from build123d import *

# Parameters (mm, degrees)
SKETCH1_R           = 1.5
SKETCH1_R_2         = 1
BOSS_EXTRUDE1_DEPTH = 3
FILLET1_R           = 5
FILLET2_R           = 3.5
FILLET3_R           = 1.5


with BuildPart() as part:
    # Sketch1 → Boss-Extrude1 (new body)
    with BuildSketch(Plane.XY):
        Polygon((0, 0), (39, 0), (39, 8.610580904), (15.926488874, 8.610580904), (15.926488874, 14.070663707), (7.926488874, 14.070663707), (7.926488874, 8), (0, 8), align=None)
        with Locations((4.5, 4)):
            Circle(SKETCH1_R, mode=Mode.SUBTRACT)
        with Locations((34.5, 4)):
            Circle(SKETCH1_R, mode=Mode.SUBTRACT)
        with Locations((12.926488874, 11.070663707)):
            Circle(SKETCH1_R_2, mode=Mode.SUBTRACT)
    extrude(amount=BOSS_EXTRUDE1_DEPTH)

    # Fillet1
    # the kernel refuses this fillet: 5 mm, written as the material it takes off along each edge
    with BuildSketch(Plane(origin=(39, 8.610580904, -12.5), x_dir=(0, -1, 0), z_dir=(0, 0, 1)), Plane(origin=(39, 0, -12.5), x_dir=(-1, 0, 0), z_dir=(0, 0, 1)), Plane(origin=(0, 8, -12.5), x_dir=(1, 0, 0), z_dir=(0, 0, 1))) as fillet1_piece_1:
        with BuildLine():
            CenterArc((FILLET1_R, -FILLET1_R), FILLET1_R, 90, 90)
            Line((0, -FILLET1_R), (0, 0))
            Line((0, 0), (FILLET1_R, 0))
        make_face()
    extrude(amount=28, mode=Mode.SUBTRACT)
    with BuildSketch(Plane(origin=(0, 0, -12.5), x_dir=(1, 0, 0), z_dir=(0, 0, 1))) as fillet1_piece_2:
        with BuildLine():
            CenterArc((FILLET1_R, FILLET1_R), FILLET1_R, 180, 90)
            Line((0, FILLET1_R), (0, 0))
            Line((0, 0), (FILLET1_R, 0))
        make_face()
    extrude(amount=28, mode=Mode.SUBTRACT)

    # Fillet2
    fillet2_edges = [part.edges().sort_by_distance(p)[0] for p in [
        (7.926488874, 14.070663707, 1.5),
        (15.926488874, 14.070663707, 1.5),
    ]]
    fillet(fillet2_edges, radius=FILLET2_R)

    # Fillet3
    fillet3_edges = [part.edges().sort_by_distance(p)[0] for p in [
        (7.926488874, 8, 1.5),
        (15.926488874, 8.610580904, 1.5),
    ]]
    fillet(fillet3_edges, radius=FILLET3_R)


solid = part.part
The model under review builds one solid part; all positions refer to its coordinate system, in mm. A direction names the side the tool comes from. Round coordinates to 2 decimals unless told otherwise and drop trailing zeros. Write each loop counter-clockwise with the first axis right and the second up, starting at its lowest first coordinate (ties: lowest second). Pieces come first, ordered by that corner, then holes. Notation, with made-up numbers: (24, 52) -> (55, 52) arc R17 ccw to (55, 79) -> close; hole circle Ø5 at (-36.5, -5). An arc over 180 degrees is marked (long way). Answer as a JSON object with one key per item and string values.
1. We need section C-C on x = 19. State the section outline as (y, z) points.
Results found:
{"outline": "(0, 0) -> (8.61, 0) -> (8.61, 3) -> (0, 3) -> close"}
2. Clearance check with flat-ended pins moving along their axes: pin 1 (2.5 mm diameter, centred on x = 12.93, y = 11.07, fed in from -Z); pin 2 (0.5 mm diameter, centred on y = 10, z = 2, fed in from -X); pin 3 (1.5 mm diameter, centred on y = 2.5, z = 2, fed in from -X); pin 4 (1.1 mm diameter, centred on x = 5.5, z = 1.5, fed in from +Y). State where each tip first meets the part, or that it passes through.
Results found:
{"pin 1": "stops at z = 0", "pin 2": "stops at x = 7.93", "pin 3": "stops at x = 0.32", "pin 4": "stops at y = 8"}
3. The part is to be moulded in two halves that separate along Y. For faces 1 (the face through (13.85, 10.69, 1.48)), 2 (the face through (7.5, 8.45, 1.52)), 3 (the face through (7.926, 10, 1)), say which applies: pulls with the +Y half, pulls with the -Y half, needs draft (parallel to the pull), parting line crosses it, or undercut.
Results found:
{"face 1": "undercut", "face 2": "pulls with the +Y half", "face 3": "needs draft"}
4. Machinability: for faces 4 (the face through (19, 6, 3)), 5 (the face through (6, 8, 1)), 6 (the face through (26, 8.611, 1)), which of the approach directions +Z, -Z, +X, -X, +Y, -Y give a long, thin tool a straight path to every point of the face, cutting with its end or side? Answer none if there is none.
Results found:
{"face 4": "+Z, +X, -X, +Y, -Y", "face 5": "+Z, -Z, -X, +Y", "face 6": "+Z, -Z, +X, +Y"}
5. We need section A-A on x = 4.5. State the section outline as (y, z) points, and give its area (3 significant figures).
Results found:
{"outline": "(0.03, 0) -> (2.5, 0) -> (2.5, 3) -> (0.03, 3) -> close; (5.5, 0) -> (7.97, 0) -> (7.97, 3) -> (5.5, 3) -> close", "area": "14.8 mm^2"}
6. We need section B-B on z = 0.6. State the section outline as (x, y) points, and give its area (3 significant figures).
Results found:
{"outline": "(0.1, 4) arc R5 ccw to (5, 0) -> (34, 0) arc R5 ccw to (38.95, 4.31) arc R5 ccw to (34, 8.61) -> (17.43, 8.61) arc R1.5 cw to (15.93, 10.11) -> (15.93, 10.57) arc R3.5 ccw to (12.43, 14.07) -> (11.43, 14.07) arc R3.5 ccw to (7.93, 10.57) -> (7.93, 9.5) arc R1.5 cw to (6.43, 8) -> (5, 8) arc R5 ccw to start; hole circle Ø3 at (4.5, 4); hole circle Ø2 at (12.93, 11.07); hole circle Ø3 at (34.5, 4)", "area": "332 mm^2"}
7. We need section D-D on x = 34.5. State the section outline as (y, z) points, and give its area (3 significant figures).
Results found:
{"outline": "(0.03, 0) -> (2.5, 0) -> (2.5, 3) -> (0.03, 3) -> close; (5.5, 0) -> (8.59, 0) -> (8.59, 3) -> (5.5, 3) -> close", "area": "16.7 mm^2"}
8. To check wall thickness, follow line 1 along X through (y, z) = (3, 2.1); line 2 along Y through (x, z) = (32, 1.9); line 3 along Y through (x, z) = (4.5, 2.3). State the ranges of each line that lie inside material, in increasing order.
Results found:
{"line 1": "x = 0.42 to 3.38, 5.62 to 33.38, 35.62 to 38.58", "line 2": "y = 0 to 8.61", "line 3": "y = 0.03 to 2.5, 5.5 to 7.97"}
